Check sheet for the modelled part. Datum: model origin and axes. Units: mm. Face numbers are marked on the shaded views. A direction names the side the tool comes from. Round coordinates to 2 decimals unless told otherwise and drop trailing zeros. Order: outer loops, then holes, each group sorted by start corner. A loop starts at its lowest first (then second) coordinate and runs counter-clockwise, first axis right, second up.
```python
from build123d import *

# Parameters (mm, degrees)
SKETCH1_W               = 20
SKETCH1_H               = 25
BOSS_EXTRUDE1_DEPTH     = 2
SKETCH4_W               = 20
SKETCH4_H               = 10
BOSS_EXTRUDE3_DEPTH     = 6.5
SKETCH9_W               = 6
SKETCH9_H               = 10
BOSS_EXTRUDE6_DEPTH     = 1.3
CUT_EXTRUDE2_DEPTH      = 34.12476415
CUT_EXTRUDE2_DEPTH_BACK = 34.12476415
SKETCH5_R               = 2.3
SKETCH6_W               = 4.8
SKETCH6_H               = 4.5
BOSS_EXTRUDE4_DEPTH     = 2
SKETCH7_R               = 1
CUT_EXTRUDE3_DEPTH      = 10
SKETCH8_W               = 2
SKETCH8_H               = 15
BOSS_EXTRUDE5_DEPTH     = 6.5


with BuildPart() as part:
    # Sketch1 → Boss-Extrude1 (new body)
    with BuildSketch(Plane.XY):
        with Locations((10, 12.5)):
            Rectangle(SKETCH1_W, SKETCH1_H)
    extrude(amount=BOSS_EXTRUDE1_DEPTH)

    # Sketch4 → Boss-Extrude3 (add)
    with BuildSketch(Plane(origin=(0, 0, 0), x_dir=(-1, 0, 0), z_dir=(0, 0, -1))):
        with Locations((-10, 20)):
            Rectangle(SKETCH4_W, SKETCH4_H)
    extrude(amount=BOSS_EXTRUDE3_DEPTH)

    # Sketch9 → Boss-Extrude6 (add)
    with BuildSketch(Plane(origin=(0, 0, -6.5), x_dir=(-1, 0, 0), z_dir=(0, 0, -1))):
        with Locations((-10, 20)):
            Rectangle(SKETCH9_W, SKETCH9_H)
    extrude(amount=BOSS_EXTRUDE6_DEPTH)

    # Sketch5 → Cut-Extrude2 (cut, two sides: drawn at the far end of the back side and taken through both)
    with BuildSketch(Plane(origin=(0, 0, -6.5), x_dir=(-1, 0, 0), z_dir=(0, 0, -1)).offset(-CUT_EXTRUDE2_DEPTH_BACK)):
        with Locations((-10, 20)):
            Circle(SKETCH5_R)
    extrude(amount=CUT_EXTRUDE2_DEPTH + CUT_EXTRUDE2_DEPTH_BACK, mode=Mode.SUBTRACT)

    # Sketch6 → Boss-Extrude4 (add)
    with BuildSketch(Plane.XY.offset(2)):
        with Locations((-2.4, 2.25)):
            Rectangle(SKETCH6_W, SKETCH6_H)
    extrude(amount=-BOSS_EXTRUDE4_DEPTH)

    # Sketch7 → Cut-Extrude3 (cut)
    with BuildSketch(Plane(origin=(0, 0, 0), x_dir=(-1, 0, 0), z_dir=(0, 0, -1))):
        with Locations((1.5, 2.25)):
            Circle(SKETCH7_R)
        with Locations((-8.5, 2.25)):
            Circle(SKETCH7_R)
    extrude(amount=-CUT_EXTRUDE3_DEPTH, mode=Mode.SUBTRACT)

    # Sketch8 → Boss-Extrude5 (add)
    with BuildSketch(Plane(origin=(0, 0, 0), x_dir=(-1, 0, 0), z_dir=(0, 0, -1))):
        with Locations((-19, 7.5)):
            Rectangle(SKETCH8_W, SKETCH8_H)
    extrude(amount=BOSS_EXTRUDE5_DEPTH)


solid = part.part
```
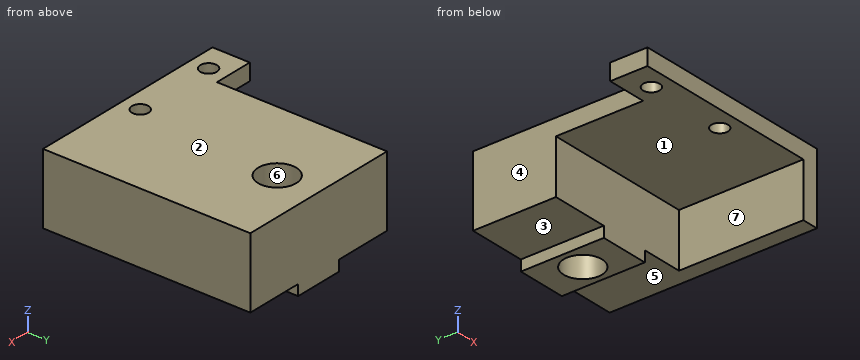
Item 1: Scan lines: line 1 along Y through (x, z) = (10, -4.5); line 2 along Y through (x, z) = (8.5, 1.55); line 3 along X through (y, z) = (1.5, 1.25). Record each from-to range of solid material in increasing order.
Answer:
line 1: y = 15 to 17.7, 22.3 to 25
line 2: y = 0 to 1.25, 3.25 to 18.26, 21.74 to 25
line 3: x = -4.8 to -2.16, -0.84 to 7.84, 9.16 to 20
Item 2: Sectioned sample at C-C (z = -3.75). Record the cut outline in (x, y).
Answer:
outline: (0, 15) - (18, 15) - (18, 0) - (20, 0) - (20, 25) - (0, 25) - close; hole circle Ø4.6 at (10, 20)
Item 3: Go/stop test with flat-tipped pins: P1, Ø2.5, axis at y = 15.5, z = -4.5, coming from the -X side; P2, Ø1.2, axis at x = 8.5, y = 2.25, coming from the -Z side; P3, Ø4, axis at x = 7, y = 5, coming from the -Z side; P4, Ø2, axis at x = 4.5, y = 20, coming from the -Z side. Record where each tip stops, or that it passes through.
Answer:
P1: stops at x = 0
P2: passes through
P3: stops at z = 0
P4: stops at z = -6.5
Item 4: Access from +Z, -Z, +X, -X, +Y, -Y to the whole of each face (thin tool, end or side, straight path). Record for the marked faces 1, 2, 3 and 4.
Answer:
face 1: -Z, -X, -Y
face 2: +Z, +X, -X, +Y, -Y
face 3: -Z, -X, +Y, -Y
face 4: +Z, -Z, -X, +Y
Item 5: Sectioned sample at B-B (x = -1.5). Record the cut outline in (y, z), and give its area (3 significant figures).
Answer:
outline: (0, 0) - (1.25, 0) - (1.25, 2) - (0, 2) - close; (3.25, 0) - (4.5, 0) - (4.5, 2) - (3.25, 2) - close
area: 5.00 mm2
Item 6: Release check for a two-part mould opening along X. For the marked faces 5, 6 and 7 record: released by +X, released by -X, zero draft, split by the parting line, or undercut.
Answer:
face 5: zero draft
face 6: undercut
face 7: released by -X
Item 7: Sectioned sample at A-A (y = 2.25). Record the cut outline in (x, z), and give its area (3 significant figures).
Answer:
outline: (-4.8, 0) - (-2.5, 0) - (-2.5, 2) - (-4.8, 2) - close; (-0.5, 0) - (7.5, 0) - (7.5, 2) - (-0.5, 2) - close; (9.5, 0) - (18, 0) - (18, -6.5) - (20, -6.5) - (20, 2) - (9.5, 2) - close
area: 54.6 mm2
Item 8: Sectioned sample at D-D (y = 20). Record the cut outline in (x, z).
Answer:
outline: (0, -6.5) - (7, -6.5) - (7, -7.8) - (7.7, -7.8) - (7.7, 2) - (0, 2) - close; (12.3, -7.8) - (13, -7.8) - (13, -6.5) - (20, -6.5) - (20, 2) - (12.3, 2) - close
